Autodesk Inventor part; units mm, degrees
ref_plane "YZ Plane" through (0, 0, 0) normal (1, 0, 0) x (0, 1, 0)
ref_plane "XZ Plane" through (0, 0, 0) normal (0, 1, 0) x (-1, 0, 0)
ref_plane "XY Plane" through (0, 0, 0) normal (0, 0, 1) x (1, 0, 0)
sketch "Sketch1" plane through (0, 0, 0) normal (0, 1, 0) x (-1, 0, 0)
  line L0 (-40, 17.5) -> (40, 17.5)
  line L1 (40, 17.5) -> (40, -17.5)
  line L2 (40, -17.5) -> (-40, -17.5)
  line L3 (-40, -17.5) -> (-40, 17.5)
  line L4 (-40, 17.5) -> (40, -17.5) construction
  line L5 (40, 17.5) -> (-40, -17.5) construction
  point P0 (0, 0)
  point P1 (0, 0)
  dimension "d10" = 80
  dimension "d11" = 35
extrude "Extrusion3" add sketch "Sketch1" along normal mid plane 4.7
sketch "Sketch3" plane through (0, 2.35, 0) normal (0, 1, 0) x (1, 0, 0)
  line L0 (-40, 17.5) -> (-40, -17.5)
  circle A0 centre (-28.75, 0) radius 4.5
  circle A1 centre (0, 0) radius 17.5
  line L1 (40, -17.5) -> (40, 17.5)
  circle A2 centre (28.75, 0) radius 4.5
  line L2 (17.5, 0) -> (17.5, -17.5)
  line L3 (-40, -17.5) -> (40, -17.5)
  dimension "d18" = 35
  dimension "d15" = 9
  dimension "d17" = 9
  dimension "d19" = 22.5
  dimension "d20" = 11.25
  dimension "d21" = 11.25
extrude "Extrusion4" cut sketch "Sketch3" against normal through all contours A0 | A2
fillet "Fillet1" radius 4 4 edges at (-40, 0, 17.5) (40, 0, 17.5) (40, 0, -17.5) (-40, 0, -17.5)
equation "\"d15\" = d17"
equation "\"d20\" = 0.5 * d19"
equation "\"d21\" = d20"
properties part number "SP11V1 Planchuela Baranda" material "Acero, carbono"
Could you check a few things on this model? Use its own coordinates, in mm. Give positions to 0.01 mm unless a question says otherwise; leave off trailing zeros. Order: outer loops, then holes, each group sorted by start corner. A loop starts at its lowest first (then second) coordinate and runs counter-clockwise, first axis right, second up.
1. I need wall thicknesses on L1, parallel to X at y = -0.4, z = 0; L2, parallel to Z at x = -28.75, y = 0.35; L3, parallel to Z at x = 30.5, y = -0.1. Which ranges of each line are inside material? Lowest first, please.
Answers below:
L1: x = -40 to -33.25, -24.25 to 24.25, 33.25 to 40
L2: z = -17.5 to -4.5, 4.5 to 17.5
L3: z = -17.5 to -4.15, 4.15 to 17.5
2. Thinking about a two-plate mould opening in Z: for faces 1 (the cylindrical face through (-24.458, 0.033, -1.352)), 2 (the cylindrical face through (-38.859, -0.033, -16.297)), 3 (the flat face through (-40, 0, 0)), 4 (the cylindrical face through (33.042, 0.033, -1.352)), which applies, +Z half, -Z half, draft (parallel to the pull), parting line (faces both ways), or undercut?
Answers below:
face 1: undercut
face 2: -Z half
face 3: draft
face 4: undercut
3. Suppose I cut it at C-C (y = -1.4). Write out the boundary of the cut face in (x, z).
Answers below:
outline: (-40, -13.5) arc R4 ccw to (-36, -17.5) - (36, -17.5) arc R4 ccw to (40, -13.5) - (40, 13.5) arc R4 ccw to (36, 17.5) - (-36, 17.5) arc R4 ccw to (-40, 13.5) - close; hole circle Ø9 at (-28.75, 0); hole circle Ø9 at (28.75, 0)
4. Suppose I cut it at B-B (z = 0). Write out the boundary of the cut face in (x, y), plus the area to 3 significant figures.
Answers below:
outline: (-40, -2.35) - (-33.25, -2.35) - (-33.25, 2.35) - (-40, 2.35) - close; (-24.25, -2.35) - (24.25, -2.35) - (24.25, 2.35) - (-24.25, 2.35) - close; (33.25, -2.35) - (40, -2.35) - (40, 2.35) - (33.25, 2.35) - close
area: 291 mm2
5. Suppose I cut it at A-A (x = 28.75). Write out the boundary of the cut face in (y, z), plus the area to 3 significant figures.
Answers below:
outline: (-2.35, -17.5) - (2.35, -17.5) - (2.35, -4.5) - (-2.35, -4.5) - close; (-2.35, 4.5) - (2.35, 4.5) - (2.35, 17.5) - (-2.35, 17.5) - close
area: 122 mm2
6. For pin 1 (7 mm diameter, centred on x = -28.75, z = 0, fed in from -Y), with a flat end and sliding along its axis, tell me the tip position at first contact or that it passes through.
Answers below:
pin 1: passes through
7. Suppose I cut it at D-D (x = -25). Write out the boundary of the cut face in (y, z), plus the area to 3 significant figures.
Answers below:
outline: (-2.35, -17.5) - (2.35, -17.5) - (2.35, -2.49) - (-2.35, -2.49) - close; (-2.35, 2.49) - (2.35, 2.49) - (2.35, 17.5) - (-2.35, 17.5) - close
area: 141 mm2
